Read the model definition and answer for the solid it produces. Units are mm, in the model's axes. A direction names the side the tool comes from. Give positions to 0.01 mm unless a question says otherwise; leave off trailing zeros. Write each loop counter-clockwise with the first axis right and the second up, starting at its lowest first coordinate (ties: lowest second). Pieces come first, ordered by that corner, then holes.
```python
from build123d import *

# Parameters (mm, degrees)
EXTRUDE_1_DEPTH          = 10
EXTRUDE_2_DEPTH          = 5
CUT_EXTRUDE_2_DEPTH      = 5
PATTERN_CIRCULAR_1_COUNT = 3
EXTRUDE_3_DEPTH          = 5
CUT_EXTRUDE_3_DEPTH      = 5


with BuildPart() as part:
    # Sketch 1 → Extrude 1 (new body)
    with BuildSketch(Plane.XY):
        Polygon((14.43375673, 0), (7.216878365, 12.5), (-7.216878365, 12.5), (-14.43375673, 0), (-7.216878365, -12.5), (7.216878365, -12.5), align=None)
    extrude(amount=EXTRUDE_1_DEPTH)

    # Sketch 2 → Extrude 2 (add)
    with BuildSketch(Plane(origin=(0, 0, 0), x_dir=(-1, 0, 0), z_dir=(0, 0, -1))):
        with BuildLine():
            Line((-3.122498999, 12.5), (3.122498999, 12.5))
            ThreePointArc((3.122498999, 12.5), (2.22111118, 13.066987298), (2.341874249, 14.125))
            ThreePointArc((2.341874249, 14.125), (0, 19), (-2.341874249, 14.125))
            ThreePointArc((-2.341874249, 14.125), (-2.22111118, 13.066987298), (-3.122498999, 12.5))
        make_face()
    extrude_2 = extrude(amount=-EXTRUDE_2_DEPTH)

    # Sketch 3 → Cut-Extrude 2 (cut)
    with BuildSketch(Plane(origin=(0, 0, 0), x_dir=(-1, 0, 0), z_dir=(0, 0, -1))):
        with BuildLine():
            ThreePointArc((-2.457026249, -10.890243902), (-2.352465403, -11.941726104), (-3.249615362, -12.5))
            Line((-3.249615362, -12.5), (0, -12.5))
            Line((0, -12.5), (3.249615362, -12.5))
            ThreePointArc((3.249615362, -12.5), (2.352465403, -11.941726104), (2.457026249, -10.890243902))
            ThreePointArc((2.457026249, -10.890243902), (0, -5.9), (-2.457026249, -10.890243902))
        make_face()
    cut_extrude_2 = extrude(amount=-CUT_EXTRUDE_2_DEPTH, mode=Mode.SUBTRACT)

    # Pattern Circular 1: Extrude 2, Cut-Extrude 2 ×3 about axis
    pattern_circular_1_axis = Axis((0, 0, 0), (0, 0, 1))
    add([extrude_2.rotate(pattern_circular_1_axis, i * 360 / PATTERN_CIRCULAR_1_COUNT) for i in range(1, PATTERN_CIRCULAR_1_COUNT)])
    add([cut_extrude_2.rotate(pattern_circular_1_axis, i * 360 / PATTERN_CIRCULAR_1_COUNT) for i in range(1, PATTERN_CIRCULAR_1_COUNT)], mode=Mode.SUBTRACT)

    # Sketch 5 → Extrude 3 (add)
    with BuildSketch(Plane.XY.offset(10)):
        with BuildLine():
            Line((7.216878365, -12.5), (9.200509866, -9.064249456))
            ThreePointArc((9.200509866, -9.064249456), (9.16560547, -8.008157853), (8.202714748, -7.572969101))
            ThreePointArc((8.202714748, -7.572969101), (5.109549882, -2.95), (10.659740998, -3.317274802))
            ThreePointArc((10.659740998, -3.317274802), (11.518070873, -3.933568252), (12.450125228, -3.435750544))
            Line((12.450125228, -3.435750544), (14.43375673, 0))
            Line((14.43375673, 0), (12.386567047, 3.545836543))
            ThreePointArc((12.386567047, 3.545836543), (12.426898541, 4.609954942), (13.403545953, 5.034377408))
            ThreePointArc((13.403545953, 5.034377408), (16.454482672, 9.5), (11.061671704, 9.090622592))
            ThreePointArc((11.061671704, 9.090622592), (10.205787361, 8.457032356), (9.264068048, 8.954163457))
            Line((9.264068048, 8.954163457), (7.216878365, 12.5))
            Line((7.216878365, 12.5), (3.249615362, 12.5))
            ThreePointArc((3.249615362, 12.5), (2.352465403, 11.941726104), (2.457026249, 10.890243902))
            ThreePointArc((2.457026249, 10.890243902), (0, 5.9), (-2.457026249, 10.890243902))
            ThreePointArc((-2.457026249, 10.890243902), (-2.352465403, 11.941726104), (-3.249615362, 12.5))
            Line((-3.249615362, 12.5), (-7.216878365, 12.5))
            Line((-7.216878365, 12.5), (-9.264068048, 8.954163457))
            ThreePointArc((-9.264068048, 8.954163457), (-10.205787361, 8.457032356), (-11.061671704, 9.090622592))
            ThreePointArc((-11.061671704, 9.090622592), (-16.454482672, 9.5), (-13.403545953, 5.034377408))
            ThreePointArc((-13.403545953, 5.034377408), (-12.426898541, 4.609954942), (-12.386567047, 3.545836543))
            Line((-12.386567047, 3.545836543), (-14.43375673, 0))
            Line((-14.43375673, 0), (-12.450125228, -3.435750544))
            ThreePointArc((-12.450125228, -3.435750544), (-11.518070873, -3.933568252), (-10.659740998, -3.317274802))
            ThreePointArc((-10.659740998, -3.317274802), (-5.109549882, -2.95), (-8.202714748, -7.572969101))
            ThreePointArc((-8.202714748, -7.572969101), (-9.16560547, -8.008157853), (-9.200509866, -9.064249456))
            Line((-9.200509866, -9.064249456), (-7.216878365, -12.5))
            Line((-7.216878365, -12.5), (-3.122498999, -12.5))
            ThreePointArc((-3.122498999, -12.5), (-2.22111118, -13.066987298), (-2.341874249, -14.125))
            ThreePointArc((-2.341874249, -14.125), (0, -19), (2.341874249, -14.125))
            ThreePointArc((2.341874249, -14.125), (2.22111118, -13.066987298), (3.122498999, -12.5))
            Line((3.122498999, -12.5), (7.216878365, -12.5))
        make_face()
    extrude(amount=-EXTRUDE_3_DEPTH)

    # Sketch 6 → Cut-Extrude 3 (cut)
    with BuildSketch(Plane.XY.offset(10)):
        Polygon((26.179583505, 0.365011735), (12.773682317, 22.854690243), (-13.405901188, 22.489678508), (-26.179583505, -0.365011735), (-12.773682317, -22.854690243), (13.405901188, -22.489678508), align=None)
        with BuildLine():
            Line((7.216878365, -12.5), (9.200509866, -9.064249456))
            ThreePointArc((9.200509866, -9.064249456), (9.16560547, -8.008157853), (8.202714748, -7.572969101))
            ThreePointArc((8.202714748, -7.572969101), (5.109549882, -2.95), (10.659740998, -3.317274802))
            ThreePointArc((10.659740998, -3.317274802), (11.518070873, -3.933568252), (12.450125228, -3.435750544))
            Line((12.450125228, -3.435750544), (14.43375673, 0))
            Line((14.43375673, 0), (12.386567047, 3.545836543))
            ThreePointArc((12.386567047, 3.545836543), (12.426898541, 4.609954942), (13.403545953, 5.034377408))
            ThreePointArc((13.403545953, 5.034377408), (16.454482672, 9.5), (11.061671704, 9.090622592))
            ThreePointArc((11.061671704, 9.090622592), (10.205787361, 8.457032356), (9.264068048, 8.954163457))
            Line((9.264068048, 8.954163457), (7.216878365, 12.5))
            Line((7.216878365, 12.5), (3.249615362, 12.5))
            ThreePointArc((3.249615362, 12.5), (2.352465403, 11.941726104), (2.457026249, 10.890243902))
            ThreePointArc((2.457026249, 10.890243902), (0, 5.9), (-2.457026249, 10.890243902))
            ThreePointArc((-2.457026249, 10.890243902), (-2.352465403, 11.941726104), (-3.249615362, 12.5))
            Line((-3.249615362, 12.5), (-7.216878365, 12.5))
            Line((-7.216878365, 12.5), (-9.264068048, 8.954163457))
            ThreePointArc((-9.264068048, 8.954163457), (-10.205787361, 8.457032356), (-11.061671704, 9.090622592))
            ThreePointArc((-11.061671704, 9.090622592), (-16.454482672, 9.5), (-13.403545953, 5.034377408))
            ThreePointArc((-13.403545953, 5.034377408), (-12.426898541, 4.609954942), (-12.386567047, 3.545836543))
            Line((-12.386567047, 3.545836543), (-14.43375673, 0))
            Line((-14.43375673, 0), (-12.450125228, -3.435750544))
            ThreePointArc((-12.450125228, -3.435750544), (-11.518070873, -3.933568252), (-10.659740998, -3.317274802))
            ThreePointArc((-10.659740998, -3.317274802), (-5.109549882, -2.95), (-8.202714748, -7.572969101))
            ThreePointArc((-8.202714748, -7.572969101), (-9.16560547, -8.008157853), (-9.200509866, -9.064249456))
            Line((-9.200509866, -9.064249456), (-7.216878365, -12.5))
            Line((-7.216878365, -12.5), (-3.122498999, -12.5))
            ThreePointArc((-3.122498999, -12.5), (-2.22111118, -13.066987298), (-2.341874249, -14.125))
            ThreePointArc((-2.341874249, -14.125), (0, -19), (2.341874249, -14.125))
            ThreePointArc((2.341874249, -14.125), (2.22111118, -13.066987298), (3.122498999, -12.5))
            Line((3.122498999, -12.5), (7.216878365, -12.5))
        make_face(mode=Mode.SUBTRACT)
    extrude(amount=-CUT_EXTRUDE_3_DEPTH, mode=Mode.SUBTRACT)


solid = part.part
```
Item 1: Which of the six approach directions +Z, -Z, +X, -X, +Y, -Y give full straight-line access (tool end or side, diameter ignored) to faces 1 (the flat face through (-13.396, 1.798, 4.93)), 2 (the cylindrical face through (-2.346, 11.928, 7.535)), 3 (the cylindrical face through (5.159, 2.867, 2.465)), 4 (the flat face through (-5, -12.5, 5))?
Result set:
face 1: +Z, -Z, -X
face 2: +Z
face 3: -Z
face 4: +Z, -Z, -X, -Y
Item 2: Determine the mould class of faces 5 (the flat face through (5, 12.5, 5)), 6 (the flat face through (-13.424, -1.748, 4.93)), 7 (the flat face through (8.2, -10.8, 4.9)) for opening direction Y: pulls with the +Y half, pulls with the -Y half, needs draft (parallel to the pull), parting line crosses it, or undercut.
Result set:
face 5: pulls with the +Y half
face 6: undercut
face 7: pulls with the -Y half
Item 3: Section C-C (y = -4.5) is taken. Write down the section's boundary in (x, z), and give its area (3 significant figures).
Result set:
outline: (-12.36, 0) - (12.36, 0) - (12.36, 5) - (4.69, 5) - (4.69, 10) - (-4.69, 10) - (-4.69, 5) - (-12.36, 5) - close
area: 171 mm2
Item 4: Section D-D (y = -16) is taken. Write down the section's boundary in (x, z), and give its area (3 significant figures).
Result set:
outline: (-3, 5) - (3, 5) - (3, 10) - (-3, 10) - close
area: 30.0 mm2
Item 5: Find the intervals of material crossed by line 1 along X through (y, z) = (10.5, 9.25); line 2 along X through (y, z) = (9, 8.55); line 3 along Z through (x, y) = (-6.5, -4.5), in increasing order.
Result set:
line 1: x = -15.51 to -12.2, -8.37 to -2.71, 2.71 to 8.37, 12.2 to 15.51
line 2: x = -16.68 to -11.02, -9.24 to -3.1, 3.1 to 9.24, 11.02 to 16.68
line 3: z = 0 to 5
Item 6: Section A-A (x = 0) is taken. Write down the section's boundary in (y, z), and give its area (3 significant figures).
Result set:
outline: (-19, 5) - (-5.9, 5) - (-5.9, 0) - (19, 0) - (19, 5) - (5.9, 5) - (5.9, 10) - (-19, 10) - close
area: 249 mm2
Item 7: Each of these flat-tipped pins is pushed along its axis until it touches: pin 1 Ø3 at (x, z) = (5.5, 8) entering from -Y; pin 2 Ø5 at (x, y) = (-13.5, 7.5) entering from -Z; pin 3 Ø1.2 at (x, z) = (4, 6) entering from +Y. Where does it stop, or does it pass through?
Result set:
pin 1: stops at y = -12.5
pin 2: stops at z = 5
pin 3: stops at y = 12.5
